from build123d import *

# Parameters (mm, degrees)
F1_DEPTH = 63.5
F2_DEPTH = 25.4
F3_DEPTH = 7.9375
F0_W     = 25.47402
F0_H     = 19.05
F5_R     = 6.35


with BuildPart() as f1:
    # F0 (on Front) → F1 (new body, symmetric)
    with BuildSketch(Plane.XZ):
        Polygon((22.225, 9.525), (-41.275, 9.525), (-41.275, -9.525), (41.275, -9.525), (41.275, 9.525), align=None)
    extrude(amount=F1_DEPTH, both=True)

    # F0 (on Front) → F2 (join, symmetric)
    with BuildSketch(Plane.XZ):
        with BuildLine():
            Line((22.225, 26.99499), (22.225, 9.525))
            Line((22.225, 9.525), (41.275, 9.525))
            Line((41.275, 9.525), (41.275, 26.99499))
            ThreePointArc((41.275, 26.99499), (45.926206, 38.223994), (57.15521, 42.8752))
            Line((57.15521, 42.8752), (60.325, 42.8752))
            Line((60.325, 42.8752), (60.325, 61.9252))
            Line((60.325, 61.9252), (57.15521, 61.9252))
            add(Edge.make_bspline(
                [(56.465119, 61.918383), (56.694879, 61.920891), (56.92491, 61.923164), (57.15521, 61.9252)],
                knots=[111.059822, 111.059822, 111.059822, 111.059822, 111.509135, 111.509135, 111.509135, 111.509135], degree=3))
            ThreePointArc((56.465119, 61.918383), (32.213031, 51.449178), (22.225, 26.99499))
        make_face()
    extrude(amount=F2_DEPTH, both=True)

    # F0 (on Front) → F3 (join, symmetric)
    with BuildSketch(Plane.XZ):
        with BuildLine():
            add(Edge.make_bspline(
                [(-41.275, 9.525), (-40.571277, 46.227381), (-0.326284, 61.298251), (56.465119, 61.918383)],
                knots=[0, 0, 0, 0, 111.059822, 111.059822, 111.059822, 111.059822], degree=3))
            Line((-41.275, 9.525), (22.225, 9.525))
            Line((22.225, 9.525), (22.225, 26.99499))
            ThreePointArc((22.225, 26.99499), (32.213031, 51.449178), (56.465119, 61.918383))
        make_face()
    extrude(amount=F3_DEPTH, both=True)

    # F0 (on Front) → F4 (revolve)
    with BuildSketch(Plane.XZ):
        with Locations((73.06201, 52.4002)):
            Rectangle(F0_W, F0_H)
    revolve(axis=Axis((60.325, 0, 52.3875), (0, 0, 1)))

    # F5
    f5_edges = [f1.edges().sort_by_distance(p)[0] for p in [
        (41.275, 63.5, 0),
        (-41.275, 63.5, 0),
        (41.275, -63.5, 0),
        (-41.275, -63.5, 0),
    ]]
    fillet(f5_edges, radius=F5_R)


solid = f1.part
Source: CAD feature listing. Evaluate the final solid. Frame: model axes, mm. A direction names the side the tool comes from. Round coordinates to 2 decimals unless told otherwise and drop trailing zeros. Loops run counter-clockwise (first coordinate to the right, second up) from the corner with the lowest first, then second, coordinate; pieces in that order, holes last. Notation, with made-up numbers: M 71.25,-6.5 L 92.25,-6.5 A38 ccw 92.25,32.5 Z; hole C 42.5,14 d4. An arc over 180 degrees is marked long. Return JSON: item names as keys, results as strings. Group by question number.
1. Pin query (flat end, axial travel): pin 1 (18 mm diameter, centred on x = 47, z = 34, fed in from -Y); pin 2 (5 mm diameter, centred on x = 39.5, z = 11, fed in from -Y); pin 3 (18 mm diameter, centred on x = 47.5, z = 41, fed in from +Y). Return the tip coordinate at first contact, or that it passes through.
2. Reachability of faces 1 (the face through (34.85, 0.17, 61.55)), 2 (the face through (41.275, -1, 4)), 3 (the face through (-2, -7.938, 30)), 4 (the face through (22.225, 17, 18)) from +Z, -Z, +X, -X, +Y, -Y: full face, straight path, thin tool, end or side. Return the list, or none.
3. Section query A-A on z = 0. Output: boundary loops of the cut face in (x, y) (3 decimals), and give its area (3 significant figures).
4. Section query B-B on y = 23.5. Output: boundary loops of the cut face in (x, z) (3 decimals), and give its area (3 significant figures).
5. Section query C-C on y = -34.5. Output: boundary loops of the cut face in (x, z) (3 decimals).
6. Material intervals for line 1 along Y through (x, z) = (1, 38); line 2 along Z through (x, y) = (-19.5, -38) (3 decimals); line 3 along Y through (x, z) = (29, 22), sorted ascending. Write a range as from..to.
Checks:
{
 "1": {"pin 1": "stops at y = -25.4", "pin 2": "stops at y = -62.96", "pin 3": "stops at y = 25.4"},
 "2": {"face 1": "+Z, -X", "face 2": "-Z, +X, +Y, -Y", "face 3": "+Z, -X, -Y", "face 4": "+Z, -X, +Y"},
 "3": {"outline": "M -41.275,-57.15 A6.35 ccw -34.925,-63.5 L 34.925,-63.5 A6.35 ccw 41.275,-57.15 L 41.275,57.15 A6.35 ccw 34.925,63.5 L -34.925,63.5 A6.35 ccw -41.275,57.15 Z", "area": "10,400 mm²"},
 "4": {"outline": "M -41.275,-9.525 L 41.275,-9.525 L 41.275,26.995 A15.88 cw 57.155,42.875 L 70.157,42.875 L 70.157,61.925 L 50.493,61.925 L 50.493,61.284 A34.93 ccw 22.225,26.995 L 22.225,9.525 L -41.275,9.525 Z", "area": "2,910 mm²"},
 "5": {"outline": "M -41.275,-9.525 L 41.275,-9.525 L 41.275,9.525 L -41.275,9.525 Z"},
 "6": {"line 1": "y = -7.94..7.94", "line 2": "z = -9.525..9.525", "line 3": "y = -25.4..25.4"}
}
